```python
from build123d import *

# Parameters (mm, degrees)
RESSALTO_EXTRUS_O1_DEPTH = 8
ESBO_O2_W                = 32.3
ESBO_O2_H                = 16.047818473
CORTE_EXTRUS_O1_DEPTH    = 149.344709352
ESBO_O3_W                = 8
ESBO_O3_H                = 47.952181527
RESSALTO_EXTRUS_O2_DEPTH = 8
FURO_COM_FOLGA_DE_M81_D  = 9
FURO_COM_FOLGA_DE_M61_D  = 6.6
FILETE1_R                = 10
ESBO_O9_W                = 10.453941956
ESBO_O9_H                = 5.226970978
CORTE_EXTRUS_O2_DEPTH    = 142.026976627


with BuildPart() as part:
    # Esboço1 → Ressalto-extrusão1 (new body)
    with BuildSketch(Plane(origin=(0, 0, 0), x_dir=(0, 0, -1), z_dir=(1, 0, 0))):
        Polygon((28, 74), (39.129876604, 32.462735031), (128.320508076, 0), (33.320508076, 0), (16, 10), (0, 10), (0, 74), align=None)
    extrude(amount=RESSALTO_EXTRUS_O1_DEPTH)

    # Esboço2 → Corte-extrusão1 (cut, through all)
    with BuildSketch(Plane(origin=(8, 0, 0), x_dir=(0, 0, -1), z_dir=(1, 0, 0))):
        with Locations((16.15, 65.976090763)):
            Rectangle(ESBO_O2_W, ESBO_O2_H)
    extrude(amount=-CORTE_EXTRUS_O1_DEPTH, mode=Mode.SUBTRACT)

    # Esboço3 → Ressalto-extrusão2 (add)
    with BuildSketch(Plane(origin=(8, 0, 0), x_dir=(0, 0, -1), z_dir=(1, 0, 0))):
        with Locations((-4, 33.976090763)):
            Rectangle(ESBO_O3_W, ESBO_O3_H)
    extrude(amount=-RESSALTO_EXTRUS_O2_DEPTH)

    # Furo com folga de M81 (through all)
    with Locations(Plane.ZY):
        with Locations((-4, 45.952181527), (-12, 22)):
            Hole(FURO_COM_FOLGA_DE_M81_D / 2)

    # Furo com folga de M61 (through all)
    with Locations(Plane(origin=(8, 0, 0), x_dir=(0, 0, -1), z_dir=(1, 0, 0))):
        with Locations((26.161384096, 49.952181527), (30.043669773, 35.463294133), (33.925955449, 20.974406739)):
            Hole(FURO_COM_FOLGA_DE_M61_D / 2)

    # Filete1
    filete1_edges = [part.edges().sort_by_distance(p)[0] for p in [
        (4, 32.462735031, -39.129876604),
    ]]
    fillet(filete1_edges, radius=FILETE1_R)

    # Esboço9 → Corte-extrusão2 (cut, through all)
    with BuildSketch(Plane(origin=(8, 0, 0), x_dir=(0, 0, -1), z_dir=(1, 0, 0))):
        with Locations((47.673601146, 13.077387372)):
            Rectangle(ESBO_O9_W, ESBO_O9_H)
    extrude(amount=-CORTE_EXTRUS_O2_DEPTH, mode=Mode.SUBTRACT)


solid = part.part
```
Could you check a few things on this model? Use its own coordinates, in mm. A direction names the side the tool comes from. Round coordinates to 2 decimals unless told otherwise and drop trailing zeros. Loops run counter-clockwise (first coordinate to the right, second up) from the corner with the lowest first, then second, coordinate; pieces in that order, holes last. Notation, with made-up numbers: (6, 78) -> (51, 78) arc R24 cw to (51, 99) -> close; hole circle Ø3 at (21.5, 71). An arc over 180 degrees is marked (long way). Put each result on its own line as item: value.
Q1. I want a section at C-C on z = -91.5. Write out the boundary of the cut face in (x, y), and give its area (3 significant figures).
Checks:
outline: (0, 0) -> (8, 0) -> (8, 13.4) -> (0, 13.4) -> close
area: 107 mm2
Q2. Which directions (+Z, -Z, +X, -X, +Y, -Y) give clear straight access to the entire face, cutting with the end or side of a thin tool? Please do faces 1 (the flat face through (8, 23, -29)), 2 (the flat face through (4, 13, -52.901)), 3 (the flat face through (4, 10, -4)).
Checks:
face 1: +Z, -Z, +X, +Y, -Y
face 2: +X, -X
face 3: +Z, +X, -X, -Y
Q3. For pin 1 Ø6 at (y, z) = (20.97, -33.93) entering from -X; pin 2 Ø2.5 at (x, z) = (3.5, -7) entering from -Y; pin 3 Ø2 at (x, z) = (7, -87) entering from +Y; pin 4 Ø4 at (x, z) = (6, -47.5) entering from +Y, each with a flat end and sliding along its axis, tell me the tip position at first contact or that it passes through.
Checks:
pin 1: through
pin 2: y = 10
pin 3: y = 15.4
pin 4: y = 30.14
Q4. I want a section at A-A on z = -12. Write out the boundary of the cut face in (x, y), and give its area (3 significant figures).
Checks:
outline: (0, 10) -> (8, 10) -> (8, 17.5) -> (0, 17.5) -> close; (0, 26.5) -> (8, 26.5) -> (8, 57.95) -> (0, 57.95) -> close
area: 312 mm2
Q5. Thinking about a two-plate mould opening in Y: for faces 4 (the flat face through (4, 57.952, -12)), 5 (the flat face through (4, 13, -42.447)), 6 (the flat face through (3.94, 4.93, -24.78)), 7 (the flat face through (0, 23, -29)), which applies, pulls with the +Y half, pulls with the -Y half, needs draft (parallel to the pull), parting line crosses it, or undercut?
Checks:
face 4: pulls with the +Y half
face 5: undercut
face 6: pulls with the -Y half
face 7: needs draft
Q6. Please list where these lines run through material, in increasing order: line 1 (Y direction, x = 3.5, z = -12); line 2 (Y direction, x = 1.75, z = -4); line 3 (Z direction, x = 3, y = 47.5). Write a range as from..to.
Checks:
line 1: 10..17.5, 26.5..57.95
line 2: 10..41.45, 50.45..57.95
line 3: -35.1..-28.37, -23.95..-8.23, 0.23..8
Q7. I want a section at D-D on z = -110. Write out the boundary of the cut face in (x, y).
Checks:
outline: (0, 0) -> (8, 0) -> (8, 6.67) -> (0, 6.67) -> close
Q8. I want a section at B-B on x = 6.75. Write out the boundary of the cut face in (y, z), and give its area (3 significant figures).
Checks:
outline: (0, -128.32) -> (30.68, -44.02) arc R10 cw to (37.49, -37.78) -> (57.95, -32.3) -> (57.95, 8) -> (10, 8) -> (10, -16) -> (0, -33.32) -> close; hole (10.46, -52.9) -> (15.69, -52.9) -> (15.69, -42.45) -> (10.46, -42.45) -> close; hole circle Ø9 at (22, -12); hole circle Ø6.6 at (20.97, -33.93); hole circle Ø6.6 at (35.46, -30.04); hole circle Ø9 at (45.95, -4); hole circle Ø6.6 at (49.95, -26.16)
area: 3,480 mm2
